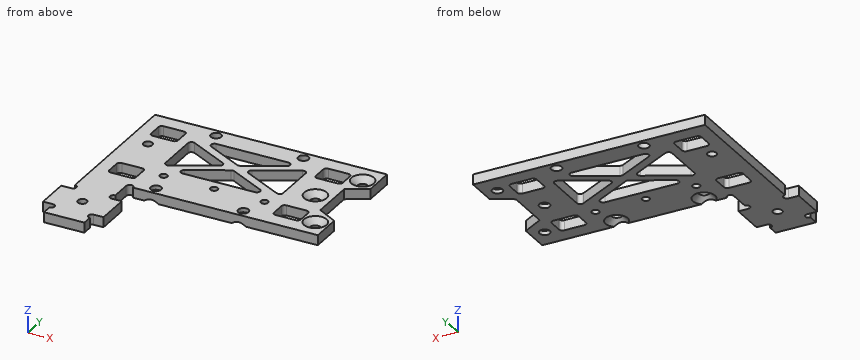
```python
from build123d import *

# Parameters (mm, degrees)
SKETCH_1_R                  = 1.55
SKETCH_1_W                  = 8
SKETCH_1_H                  = 6
EXTRUDE_1_DEPTH             = 3
HOLE_WIZARD_M3_1_AT_2_COUNT = 2
HOLE_WIZARD_M3_1_AT_2_PITCH = 14.76482306
HOLE_WIZARD_M3_1_AT_3_COUNT = 2
HOLE_WIZARD_M3_1_AT_3_PITCH = 26
SKETCH_3_R                  = 1.1
SKETCH_3_R_2                = 1.35
CUT_EXTRUDE_1_DEPTH         = 42.258332492
SKETCH_4_R                  = 1.35
EXTRUDE_2_DEPTH             = 3
SKETCH_5_R                  = 1
CUT_EXTRUDE_2_DEPTH         = 56.724770076
FILLET_1_R                  = 1
HOLE_WIZARD_1_AT_2_COUNT    = 2
HOLE_WIZARD_1_AT_2_PITCH    = 26


with BuildPart() as part:
    # 草图1 → 凸台-拉伸1 (new body)
    with BuildSketch(Plane.XY):
        Polygon((36.5, -19), (-32.5, -19), (-32.5, 19), (36.5, 19), (36.5, 10), (30.5, 6.535898385), (30.5, -6.535898385), (36.5, -10), align=None)
        with Locations((-13, 16.5)):
            Circle(SKETCH_1_R, mode=Mode.SUBTRACT)
        with Locations((-13, -16.5)):
            Circle(SKETCH_1_R, mode=Mode.SUBTRACT)
        with Locations((13, -16.5)):
            Circle(SKETCH_1_R, mode=Mode.SUBTRACT)
        with Locations((13, 16.5)):
            Circle(SKETCH_1_R, mode=Mode.SUBTRACT)
        with Locations((32.5, -13)):
            Circle(SKETCH_1_R, mode=Mode.SUBTRACT)
        with Locations(Location((32.5, 13, 0), (0, 0, 180))):
            Circle(SKETCH_1_R, mode=Mode.SUBTRACT)
        with Locations((25.5, 0)):
            Circle(SKETCH_1_R, mode=Mode.SUBTRACT)
        with Locations((-24.5, -11.5)):
            Rectangle(SKETCH_1_W, SKETCH_1_H, mode=Mode.SUBTRACT)
        with Locations((-24.5, 11.5)):
            Rectangle(SKETCH_1_W, SKETCH_1_H, mode=Mode.SUBTRACT)
        with Locations((24.5, -11.5)):
            Rectangle(SKETCH_1_W, SKETCH_1_H, mode=Mode.SUBTRACT)
        with Locations((24.5, 11.5)):
            Rectangle(SKETCH_1_W, SKETCH_1_H, mode=Mode.SUBTRACT)
    extrude(amount=EXTRUDE_1_DEPTH)

    # 草图2 → M3 六角凹锥坑螺钉的锥形沉头孔1 (revolve, cut)
    with BuildSketch(Plane(origin=(32.5, 13, 3), x_dir=(0, -1, 0), z_dir=(1, 0, 0))):
        Polygon((0, 0), (0, 3), (1.5, 3), (1.5, 1.86), (3.36, 0), align=None)
    hole_wizard_m3_1 = revolve(axis=Axis((32.5, 13, 9.35), (0, 0, -1)), mode=Mode.SUBTRACT)

    # M3 六角凹锥坑螺钉的锥形沉头孔1 at 2: M3 六角凹锥坑螺钉的锥形沉头孔1 ×2
    with Locations(*[Vector(-0.4740998230350173, -0.8804710999221754, 0) * (i * HOLE_WIZARD_M3_1_AT_2_PITCH) for i in range(1, HOLE_WIZARD_M3_1_AT_2_COUNT)]):
        add(hole_wizard_m3_1, mode=Mode.SUBTRACT)

    # M3 六角凹锥坑螺钉的锥形沉头孔1 at 3: M3 六角凹锥坑螺钉的锥形沉头孔1 ×2
    with Locations(*[(0, -i * HOLE_WIZARD_M3_1_AT_3_PITCH, 0) for i in range(1, HOLE_WIZARD_M3_1_AT_3_COUNT)]):
        add(hole_wizard_m3_1, mode=Mode.SUBTRACT)

    # 草图3 → 切除-拉伸1 (cut, through all)
    with BuildSketch(Plane(origin=(0, 0, 0), x_dir=(-1, 0, 0), z_dir=(0, 0, -1))):
        with Locations((14.5, -9.5)):
            Circle(SKETCH_3_R)
        with Locations((-0.5, -9.5)):
            Circle(SKETCH_3_R)
        with Locations((-15.5, -9.5)):
            Circle(SKETCH_3_R)
        with Locations((26.5, 4)):
            Circle(SKETCH_3_R_2)
        Polygon((14.825100782, -6), (0, 1.836124699), (-14.825100782, -6), align=None)
        Polygon((17.5, -4.586124699), (2.674899218, 3.25), (17.5, 11.086124699), align=None)
        Polygon((0, 4.663875301), (-14.825100782, 12.5), (14.825100782, 12.5), align=None)
        Polygon((-2.674899218, 3.25), (-17.5, 11.086124699), (-17.5, -4.586124699), align=None)
    extrude(amount=-CUT_EXTRUDE_1_DEPTH, mode=Mode.SUBTRACT)

    # 草图4 → 凸台-拉伸2 (add)
    with BuildSketch(Plane(origin=(0, 0, 0), x_dir=(-1, 0, 0), z_dir=(0, 0, -1))):
        Polygon((32.5, -19), (20.5, -19), (20.5, -22), (20.5, -27), (17.5, -27), (17.5, -37), (20.5, -37), (20.5, -42), (32.5, -42), (32.5, -37), (35.5, -37), (35.5, -27), (32.5, -27), (32.5, -22), align=None)
        with Locations((26.5, -32)):
            Circle(SKETCH_4_R, mode=Mode.SUBTRACT)
    extrude(amount=-EXTRUDE_2_DEPTH)

    # 草图5 → 切除-拉伸2 (cut, through all)
    with BuildSketch(Plane(origin=(0, 0, 0), x_dir=(-1, 0, 0), z_dir=(0, 0, -1))):
        with Locations((32.5, -38)):
            Circle(SKETCH_5_R)
        with Locations((32.5, -26)):
            Circle(SKETCH_5_R)
        with Locations((19.5, -19)):
            Circle(SKETCH_5_R)
        with Locations((20.5, -38)):
            Circle(SKETCH_5_R)
        with Locations((20.5, -26)):
            Circle(SKETCH_5_R)
    extrude(amount=-CUT_EXTRUDE_2_DEPTH, mode=Mode.SUBTRACT)

    # 圆角1
    fillet_1_edges = [part.edges().sort_by_distance(p)[0] for p in [
        (-14.825100782, -6, 1.5),
        (14.825100782, -6, 1.5),
        (0, 1.836124699, 1.5),
        (2.674899218, 3.25, 1.5),
        (17.5, -4.586124699, 1.5),
        (17.5, 11.086124699, 1.5),
        (-17.5, 11.086124699, 1.5),
        (-17.5, -4.586124699, 1.5),
        (-2.674899218, 3.25, 1.5),
        (-14.825100782, 12.5, 1.5),
        (0, 4.663875301, 1.5),
        (14.825100782, 12.5, 1.5),
        (-28.5, 14.5, 1.5),
        (-28.5, 8.5, 1.5),
        (-20.5, 8.5, 1.5),
        (-20.5, 14.5, 1.5),
        (-20.5, -14.5, 1.5),
        (-20.5, -8.5, 1.5),
        (-28.5, -8.5, 1.5),
        (-28.5, -14.5, 1.5),
        (28.5, -8.5, 1.5),
        (20.5, -8.5, 1.5),
        (20.5, -14.5, 1.5),
        (28.5, -14.5, 1.5),
        (20.5, 14.5, 1.5),
        (20.5, 8.5, 1.5),
        (28.5, 8.5, 1.5),
        (28.5, 14.5, 1.5),
    ]]
    fillet(fillet_1_edges, radius=FILLET_1_R)

    # 草图6 → 打孔尺寸(%根据十字)槽沉头木螺钉的类型1 (revolve, cut)
    with BuildSketch(Plane(origin=(-13, -16.5, 0), x_dir=(0, 1, 0), z_dir=(1, 0, 0))):
        Polygon((0, 0), (0, 3), (1.55, 3), (1.55, 1.75), (3.3, 0), align=None)
    hole_wizard_1 = revolve(axis=Axis((-13, -16.5, -6.35), (0, 0, 1)), mode=Mode.SUBTRACT)

    # 打孔尺寸(%根据十字)槽沉头木螺钉的类型1 at 2: 打孔尺寸(%根据十字)槽沉头木螺钉的类型1 ×2
    with Locations(*[(i * HOLE_WIZARD_1_AT_2_PITCH, 0, 0) for i in range(1, HOLE_WIZARD_1_AT_2_COUNT)]):
        add(hole_wizard_1, mode=Mode.SUBTRACT)


solid = part.part
```
Geometry check sheet. Reference: the model listing, model coordinates, mm. Coordinates: 2 decimals unless noted, no trailing zeros. Order: outer loops, then holes, each group sorted by start corner. A loop starts at its lowest first (then second) coordinate and runs counter-clockwise, first axis right, second up. Notation, with made-up numbers: (74, 19) - (86, 19) arc R33 ccw to (86, 54) - close; hole circle Ø5 at (-37.75, -0.5). An arc over 180 degrees is marked (long way). Answer in a Markdown table with one row per item. Add a question column.
1. Material ranges on L1, parallel to Y at x = -26.5, z = 0.8; L2, parallel to X at y = 13, z = 0.5; L3, parallel to Y at x = 32.5, z = 0.8, recorded low to high. Write a range as [from, to].
2. Gauge pin test, flat ends, axial feed: pin 1 Ø3.5 at (x, y) = (32.5, -13) entering from +Z; pin 2 Ø2.5 at (x, y) = (25.5, 0) entering from -Z; pin 3 Ø0.9 at (y, z) = (-1, 2) entering from +X; pin 4 Ø1.5 at (y, z) = (3, 1.5) entering from -X. Record the tip position at first contact, or that the pin passes through.
3. Section check A-A (x = 8.5). Enter the section's corners in (y, z).
4. Section check C-C (x = 32.5). Enter the section's corners in (y, z), plus the area to 3 significant figures.
5. Section check B-B (y = -38). Enter the section's corners in (x, z).
Data:
| question | item | result |
|---|---|---|
| 1 | L1 | y = [-42, -33.35], [-30.65, -14.5], [-8.5, 2.65], [5.35, 8.5], [14.5, 19] |
| 1 | L2 | x = [-32.5, -28.5], [-20.5, 20.5], [28.5, 30.95], [34.05, 36.5] |
| 1 | L3 | y = [-19, -14.55], [-11.45, -7.69], [7.69, 11.45], [14.55, 19] |
| 2 | pin 1 | stops at z = 1.39 |
| 2 | pin 2 | passes through |
| 2 | pin 3 | stops at x = 30.5 |
| 2 | pin 4 | stops at x = -32.5 |
| 3 | outline | (-19, 0) - (-6, 0) - (-6, 3) - (-19, 3) - close; (-2.66, 0) - (0.17, 0) - (0.17, 3) - (-2.66, 3) - close; (6.33, 0) - (9.16, 0) - (9.16, 3) - (6.33, 3) - close; (12.5, 0) - (19, 0) - (19, 3) - (12.5, 3) - close |
| 4 | outline | (-19, 0) - (-14.55, 0) - (-14.55, 1.19) - (-16.36, 3) - (-19, 3) - close; (-11.45, 0) - (-7.69, 0) - (-7.69, 3) - (-9.64, 3) - (-11.45, 1.19) - close; (7.69, 0) - (11.45, 0) - (11.45, 1.19) - (9.64, 3) - (7.69, 3) - close; (14.55, 0) - (19, 0) - (19, 3) - (16.36, 3) - (14.55, 1.19) - close |
| 4 | area | 42.7 mm² |
| 5 | outline | (-31.5, 0) - (-21.5, 0) - (-21.5, 3) - (-31.5, 3) - close |
